```python
from build123d import *

# Parameters (mm, degrees)
SKETCH1_W           = 165.1
SKETCH1_H           = 292.1
BOSS_EXTRUDE1_DEPTH = 3.048
SKETCH2_R           = 10.7315
SKETCH2_R_2         = 2.0193
SKETCH2_W           = 16.173788568
SKETCH2_H           = 32.6898
SKETCH2_W_2         = 76.2
SKETCH2_H_2         = 76.2
CUT_EXTRUDE1_DEPTH  = 168.792715289
CUT_EXTRUDE2_DEPTH  = 168.792715289
SKETCH5_R           = 2.54
CUT_EXTRUDE3_DEPTH  = 168.792715289
SKETCH6_W           = 165.1
SKETCH6_H           = 5.08
CUT_EXTRUDE4_DEPTH  = 168.792715289


with BuildPart() as part:
    # Sketch1 → Boss-Extrude1 (new body)
    with BuildSketch(Plane.XY):
        Rectangle(SKETCH1_W, SKETCH1_H)
    extrude(amount=BOSS_EXTRUDE1_DEPTH)

    # Sketch2 → Cut-Extrude1 (cut, through all)
    with BuildSketch(Plane.XY):
        with Locations((0, 92.71)):
            Circle(SKETCH2_R)
        with Locations(Location((0, 38.1, 0), (0, 0, 180))):
            Circle(SKETCH2_R_2)
        with Locations(Location((0, 30.1, 0), (0, 0, 180))):
            Circle(SKETCH2_R_2)
        with Locations(Location((0, 22.1, 0), (0, 0, 180))):
            Circle(SKETCH2_R_2)
        with Locations(Location((0, 14.1, 0), (0, 0, 180))):
            Circle(SKETCH2_R_2)
        with Locations(Location((0, 6.1, 0), (0, 0, 180))):
            Circle(SKETCH2_R_2)
        with Locations(Location((0, -1.9, 0), (0, 0, 180))):
            Circle(SKETCH2_R_2)
        with Locations(Location((0, -9.9, 0), (0, 0, 180))):
            Circle(SKETCH2_R_2)
        with Locations(Location((0, -17.9, 0), (0, 0, 180))):
            Circle(SKETCH2_R_2)
        with Locations(Location((-8, 38.1, 0), (0, 0, 180))):
            Circle(SKETCH2_R_2)
        with Locations(Location((-16, 38.1, 0), (0, 0, 180))):
            Circle(SKETCH2_R_2)
        with Locations(Location((-8, 30.1, 0), (0, 0, 180))):
            Circle(SKETCH2_R_2)
        with Locations(Location((-16, 30.1, 0), (0, 0, 180))):
            Circle(SKETCH2_R_2)
        with Locations(Location((-8, 22.1, 0), (0, 0, 180))):
            Circle(SKETCH2_R_2)
        with Locations(Location((-16, 22.1, 0), (0, 0, 180))):
            Circle(SKETCH2_R_2)
        with Locations(Location((-8, 14.1, 0), (0, 0, 180))):
            Circle(SKETCH2_R_2)
        with Locations(Location((-16, 14.1, 0), (0, 0, 180))):
            Circle(SKETCH2_R_2)
        with Locations(Location((-8, 6.1, 0), (0, 0, 180))):
            Circle(SKETCH2_R_2)
        with Locations(Location((-16, 6.1, 0), (0, 0, 180))):
            Circle(SKETCH2_R_2)
        with Locations(Location((-8, -1.9, 0), (0, 0, 180))):
            Circle(SKETCH2_R_2)
        with Locations(Location((-16, -1.9, 0), (0, 0, 180))):
            Circle(SKETCH2_R_2)
        with Locations(Location((-8, -9.9, 0), (0, 0, 180))):
            Circle(SKETCH2_R_2)
        with Locations(Location((-16, -9.9, 0), (0, 0, 180))):
            Circle(SKETCH2_R_2)
        with Locations(Location((-8, -17.9, 0), (0, 0, 180))):
            Circle(SKETCH2_R_2)
        with Locations(Location((-16, -17.9, 0), (0, 0, 180))):
            Circle(SKETCH2_R_2)
        with Locations(Location((24.086894284, 14.1, 0), (0, 0, 180))):
            Circle(SKETCH2_R_2)
        with Locations(Location((8.086894284, 14.1, 0), (0, 0, 180))):
            Circle(SKETCH2_R_2)
        with Locations(Location((8.086894284, -17.9, 0), (0, 0, 180))):
            Circle(SKETCH2_R_2)
        with Locations(Location((24.086894284, 6.1, 0), (0, 0, 180))):
            Circle(SKETCH2_R_2)
        with Locations(Location((16.086894284, 6.1, 0), (0, 0, 180))):
            Circle(SKETCH2_R_2)
        with Locations(Location((8.086894284, -1.9, 0), (0, 0, 180))):
            Circle(SKETCH2_R_2)
        with Locations(Location((8.086894284, 30.1, 0), (0, 0, 180))):
            Circle(SKETCH2_R_2)
        with Locations(Location((24.086894284, 22.1, 0), (0, 0, 180))):
            Circle(SKETCH2_R_2)
        with Locations(Location((24.086894284, -1.9, 0), (0, 0, 180))):
            Circle(SKETCH2_R_2)
        with Locations(Location((24.086894284, -9.9, 0), (0, 0, 180))):
            Circle(SKETCH2_R_2)
        with Locations(Location((8.086894284, 6.1, 0), (0, 0, 180))):
            Circle(SKETCH2_R_2)
        with Locations(Location((16.086894284, 22.1, 0), (0, 0, 180))):
            Circle(SKETCH2_R_2)
        with Locations(Location((8.086894284, 22.1, 0), (0, 0, 180))):
            Circle(SKETCH2_R_2)
        with Locations(Location((8.086894284, -9.9, 0), (0, 0, 180))):
            Circle(SKETCH2_R_2)
        with Locations(Location((24.086894284, -17.9, 0), (0, 0, 180))):
            Circle(SKETCH2_R_2)
        with Locations(Location((16.086894284, 14.1, 0), (0, 0, 180))):
            Circle(SKETCH2_R_2)
        with Locations(Location((16.086894284, -17.9, 0), (0, 0, 180))):
            Circle(SKETCH2_R_2)
        with Locations(Location((16.086894284, 30.1, 0), (0, 0, 180))):
            Circle(SKETCH2_R_2)
        with Locations(Location((24.086894284, 30.1, 0), (0, 0, 180))):
            Circle(SKETCH2_R_2)
        with Locations(Location((16.086894284, -9.9, 0), (0, 0, 180))):
            Circle(SKETCH2_R_2)
        with Locations(Location((16.086894284, -1.9, 0), (0, 0, 180))):
            Circle(SKETCH2_R_2)
        with Locations(Location((16.086894284, 38.1, 0), (0, 0, 180))):
            Circle(SKETCH2_R_2)
        with Locations(Location((8.086894284, 38.1, 0), (0, 0, 180))):
            Circle(SKETCH2_R_2)
        with Locations(Location((24.086894284, 38.1, 0), (0, 0, 180))):
            Circle(SKETCH2_R_2)
        with Locations((0, 92.71)):
            Rectangle(SKETCH2_W, SKETCH2_H)
        with Locations((0, -59.69)):
            Rectangle(SKETCH2_W_2, SKETCH2_H_2)
    extrude(amount=CUT_EXTRUDE1_DEPTH, mode=Mode.SUBTRACT)

    # Sketch4 → Cut-Extrude2 (cut, through all)
    with BuildSketch(Plane.XY):
        Polygon((-12.7, 57.310847547), (-12.7, 69.85), (-82.55, 69.85), (-82.55, 146.05), (82.55, 146.05), (82.55, 69.85), (12.7, 69.85), (12.7, 57.310847547), align=None)
    extrude(amount=CUT_EXTRUDE2_DEPTH, mode=Mode.SUBTRACT)

    # Sketch5 → Cut-Extrude3 (cut, through all)
    with BuildSketch(Plane(origin=(0, 0, 0), x_dir=(-1, 0, 0), z_dir=(0, 0, -1))):
        with Locations((-44.45, -106.299)):
            Circle(SKETCH5_R)
        with Locations((-69.85, -106.299)):
            Circle(SKETCH5_R)
        with Locations((69.85, -106.299)):
            Circle(SKETCH5_R)
        with Locations((44.45, -106.299)):
            Circle(SKETCH5_R)
    extrude(amount=-CUT_EXTRUDE3_DEPTH, mode=Mode.SUBTRACT)

    # Sketch6 → Cut-Extrude4 (cut, through all)
    with BuildSketch(Plane(origin=(0, 0, 0), x_dir=(-1, 0, 0), z_dir=(0, 0, -1))):
        with Locations((0, -143.51)):
            Rectangle(SKETCH6_W, SKETCH6_H)
    extrude(amount=-CUT_EXTRUDE4_DEPTH, mode=Mode.SUBTRACT)


solid = part.part
```
Here's how the part is built. I have some questions about the finished solid (model axes, mm). Give positions to 0.01 mm unless a question says otherwise; leave off trailing zeros. Write each loop counter-clockwise with the first axis right and the second up, starting at its lowest first coordinate (ties: lowest second). Pieces come first, ordered by that corner, then holes.
(1) Imagine slicing it at B-B, the plane x = 69.85. Write out the boundary of the cut face in (y, z).
Output values:
outline: (-140.97, 0) - (-108.84, 0) - (-108.84, 3.05) - (-140.97, 3.05) - close; (-103.76, 0) - (69.85, 0) - (69.85, 3.05) - (-103.76, 3.05) - close
(2) Imagine slicing it at A-A, the plane y = -62. Write out the boundary of the cut face in (x, z).
Output values:
outline: (-82.55, 0) - (-38.1, 0) - (-38.1, 3.05) - (-82.55, 3.05) - close; (38.1, 0) - (82.55, 0) - (82.55, 3.05) - (38.1, 3.05) - close
(3) Imagine slicing it at C-C, the plane z = 2. Count the separate pieces of the cut face and the enclosed holes in it, and give its area (3 significant figures).
Output values:
separate pieces: 1
enclosed holes: 53
area: 28,000 mm2
(4) Will this pin go through, and if not, where does the flat tip stop? pin 1 (3.5 mm diameter, centred on x = 24.09, y = -9.9, fed in from -Z).
Output values:
pin 1: passes through
(5) If I drill on L1, parallel to X at y = -88, z = 1.65; L2, parallel to Y at x = 27, z = 0.45; L3, parallel to Y at x = -68.5, z = 1.8, over which ranges is the centre line in solid material (lowest first)?
Output values:
L1: x = -82.55 to -38.1, 38.1 to 82.55
L2: y = -140.97 to -97.79, -21.59 to 69.85
L3: y = -140.97 to -108.45, -104.15 to 69.85
